Verification items for the finished model (mm, model axes). Round coordinates to 2 decimals unless told otherwise and drop trailing zeros. Loops run counter-clockwise (first coordinate to the right, second up) from the corner with the lowest first, then second, coordinate; pieces in that order, holes last. Notation, with made-up numbers: (58.25, 50) -> (106.25, 50) arc R24 ccw to (106.25, 67) -> close; hole circle Ø1 at (27, 63.5). An arc over 180 degrees is marked (long way). Write item = value, one per line. Start each with the question number.
```python
from build123d import *

# Parameters (mm, degrees)
SKETCH1_R                                  = 12.7
SKETCH1_R_2                                = 11.1125
BOSS_EXTRUDE1_DEPTH                        = 716.7546056
M5_CLEARANCE_HOLE1_D                       = 5.5
SKETCH7_W                                  = 2.75
SKETCH7_H                                  = 12.7
MIRROR1_AT_THE_SECOND_PLANE_COPY_1_SKETC_W = 2.75
MIRROR1_AT_THE_SECOND_PLANE_COPY_1_SKETC_H = 12.7


with BuildPart() as part:
    # Sketch1 → Boss-Extrude1 (new, symmetric)
    with BuildSketch(Plane.XY):
        Circle(SKETCH1_R)
        Circle(SKETCH1_R_2, mode=Mode.SUBTRACT)
    extrude(amount=BOSS_EXTRUDE1_DEPTH, both=True)

    # M5 Clearance Hole1 (through all)
    with Locations(Plane(origin=(0, 12.7, 0), x_dir=(1, 0, 0), z_dir=(0, 1, 0))):
        with Locations((0, 30), (0, -30)):
            Hole(M5_CLEARANCE_HOLE1_D / 2)

    # Sketch7 → M5 Clearance Hole2 (revolve, cut)
    with BuildSketch(Plane(origin=(0, 0, 666.7546056), x_dir=(0, 0, -1), z_dir=(1, 0, 0))):
        with Locations((1.375, 6.35)):
            Rectangle(SKETCH7_W, SKETCH7_H)
    m5_clearance_hole2 = revolve(axis=Axis((0, -6.35, 666.7546056), (0, 1, 0)), mode=Mode.SUBTRACT)

    # Mirror1: M5 Clearance Hole2 across plane
    add(m5_clearance_hole2.mirror(Plane.ZX), mode=Mode.SUBTRACT)

    # Mirror1 at the second plane: M5 Clearance Hole2 across plane
    add(m5_clearance_hole2.mirror(Plane.XY), mode=Mode.SUBTRACT)

    # Mirror1 at the second plane copy 1 sketc → Mirror1 at the second plane copy 1 (revolve, cut)
    with BuildSketch(Plane(origin=(0, 0, -666.7546056), x_dir=(0, 0, 1), z_dir=(1, 0, 0))):
        with Locations((1.375, 6.35)):
            Rectangle(MIRROR1_AT_THE_SECOND_PLANE_COPY_1_SKETC_W, MIRROR1_AT_THE_SECOND_PLANE_COPY_1_SKETC_H)
    revolve(axis=Axis((0, 6.35, -666.7546056), (0, -1, 0)), mode=Mode.SUBTRACT)


solid = part.part
```
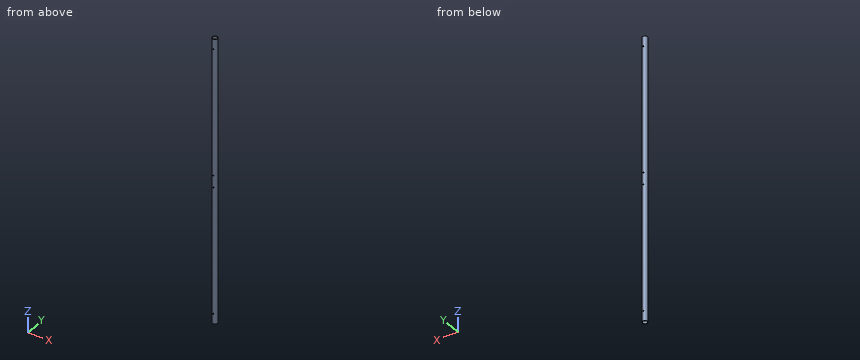
(1) Section check A-A on y = 0. Enter the section's corners in (x, z).
(2) Section check B-B on z = -278.5. Enter the section's corners in (x, y) (1 decimal), then the cut area to 3 significant figures.
(3) Depth check by flat-ended pin: pin 1 Ø1 at (y, z) = (3.5, 192) entering from +X; pin 2 Ø3 at (y, z) = (5, -532.5) entering from +X; pin 3 Ø3 at (x, z) = (-5, -157) entering from +Y; pin 4 Ø5 at (x, z) = (0, 666.75) entering from +Y. Enter the tip coordinate at first touch or a pass-through.
(4) Scan lines: line 1 (Z direction, x = 0, y = 11.6); line 2 (Y direction, x = 0.25, z = 17); line 3 (X direction, y = 2.5, z = 637). Record each from-to range of solid material in increasing order. Write a range as [from, to].
Computed values:
q1.outline = (-12.7, -716.75) -> (-11.11, -716.75) -> (-11.11, 716.75) -> (-12.7, 716.75) -> close; (11.11, -716.75) -> (12.7, -716.75) -> (12.7, 716.75) -> (11.11, 716.75) -> close
q2.outline = circle Ø25.4 at (0, 0); hole circle Ø22.2 at (0, 0)
q2.area = 119 mm²
q3.pin_1 = 12.34
q3.pin_2 = 12.21
q3.pin_3 = 12.21
q3.pin_4 = through
q4.line_1 = [-716.75, -669.5], [-664, -32.75], [-27.25, 27.25], [32.75, 664], [669.5, 716.75]
q4.line_2 = [-12.7, -11.11], [11.11, 12.7]
q4.line_3 = [-12.45, -10.83], [10.83, 12.45]
